```python
from build123d import *

# Parameters (mm, degrees)
CORNERBOSS_EXTRUDE1_DEPTH               = 20
SHELL2_T                                = -3
PUTBACKSHELLBOSS_EXTRUDE1_DEPTH         = 17
TAB_HOLES_SKETCH1_R                     = 1
TABHOLESCUT_EXTRUDE1_DEPTH              = 317.211923597
PADSKETCH3_R                            = 12
PADSKETCH3_R_2                          = 5
PADBOSS_EXTRUDE2_DEPTH                  = 10
STEPPERSHAFTHOLESKETCH4_R               = 5.1
STEPPERSHAFTHOLESKETCH4_R_2             = 1.5
STEPPERSHAFTCUT_EXTRUDE2_DEPTH          = 316.846451025
THREADEDNUTMOUNTHOLESSKETCH5_R          = 1
THREADEDNUTMOUNTHOLESCUT_EXTRUDE4_DEPTH = 10
TRPEGSKETCH1_W                          = 9.8
TRPEGSKETCH1_H                          = 13.9
TRPEGBOSS_EXTRUDE1_DEPTH                = 3.1
TRPEGCAPSKETCH2_W                       = 16
TRPEGCAPSKETCH2_H                       = 17
TRPEGCAPBOSS_EXTRUDE2_DEPTH             = 3
BOTTOMPEGHOLESKETCH3_W                  = 10
BOTTOMPEGHOLESKETCH3_H                  = 13.9
BOTTOMPEGHOLECUT_EXTRUDE1_DEPTH         = 3


with BuildPart() as part:
    # CornerrSketch1 → CornerBoss-Extrude1 (new body)
    with BuildSketch(Plane(origin=(0, 0, 0), x_dir=(1, 0, 0), z_dir=(0, 1, 0))):
        with BuildLine():
            Line((140, 220), (140, 120))
            Line((140, 120), (90, 120))
            Line((90, 120), (90, 0))
            Line((90, 0), (0, 0))
            Line((0, 0), (0, 265.825))
            ThreePointArc((0, 265.825), (17, 282.825), (34, 265.825))
            Line((34, 265.825), (34, 220))
            Line((34, 220), (140, 220))
        make_face()
    extrude(amount=CORNERBOSS_EXTRUDE1_DEPTH)

    # Shell2
    shell2_openings = [part.faces().sort_by_distance(p)[0] for p in [
        (55.952693014, 0, -131.673048366),
    ]]
    offset(amount=SHELL2_T, openings=shell2_openings, kind=Kind.INTERSECTION)

    # PutBackShellSketch2 → PutBackShellBoss-Extrude1 (add)
    with BuildSketch(Plane.XZ.offset(-17)):
        Polygon((67, -3), (87, -3), (87, -123), (137, -123), (137, -143), (67, -143), align=None)
    extrude(amount=PUTBACKSHELLBOSS_EXTRUDE1_DEPTH)

    # Tab holes-Sketch1 → TabHolesCut-Extrude1 (cut, through all)
    with BuildSketch(Plane(origin=(0, 20, 0), x_dir=(1, 0, 0), z_dir=(0, 1, 0))):
        with Locations(Location((120, 130, 0), (0, 0, 270))):
            Circle(TAB_HOLES_SKETCH1_R)
        with Locations(Location((80, 130, 0), (0, 0, 270))):
            Circle(TAB_HOLES_SKETCH1_R)
        with Locations(Location((80, 75, 0), (0, 0, 270))):
            Circle(TAB_HOLES_SKETCH1_R)
        with Locations(Location((80, 20, 0), (0, 0, 270))):
            Circle(TAB_HOLES_SKETCH1_R)
    extrude(amount=-TABHOLESCUT_EXTRUDE1_DEPTH, mode=Mode.SUBTRACT)

    # PadSketch3 → PadBoss-Extrude2 (add)
    with BuildSketch(Plane.XZ.offset(-17)):
        with Locations(Location((17, -265.825, 0), (0, 0, 90))):
            Circle(PADSKETCH3_R)
        with Locations((7, -35)):
            Circle(PADSKETCH3_R_2)
    extrude(amount=PADBOSS_EXTRUDE2_DEPTH)

    # StepperShaftHoleSketch4 → StepperShaftCut-Extrude2 (cut, through all)
    with BuildSketch(Plane.XZ.offset(-7)):
        with Locations(Location((17, -265.825, 0), (0, 0, 270))):
            Circle(STEPPERSHAFTHOLESKETCH4_R)
        with Locations(Location((7, -35, 0), (0, 0, 270))):
            Circle(STEPPERSHAFTHOLESKETCH4_R_2)
    extrude(amount=-STEPPERSHAFTCUT_EXTRUDE2_DEPTH, mode=Mode.SUBTRACT)

    # ThreadedNutMountHolesSketch5 → ThreadedNutMountHolesCut-Extrude4 (cut)
    with BuildSketch(Plane(origin=(0, 7, 0), x_dir=(-1, 0, 0), z_dir=(0, -1, 0))):
        with Locations(Location((-17, 273.825, 0), (0, 0, 90))):
            Circle(THREADEDNUTMOUNTHOLESSKETCH5_R)
        with Locations(Location((-9, 265.825, 0), (0, 0, 90))):
            Circle(THREADEDNUTMOUNTHOLESSKETCH5_R)
        with Locations(Location((-17, 257.825, 0), (0, 0, 90))):
            Circle(THREADEDNUTMOUNTHOLESSKETCH5_R)
        with Locations(Location((-25, 265.825, 0), (0, 0, 90))):
            Circle(THREADEDNUTMOUNTHOLESSKETCH5_R)
    extrude(amount=-THREADEDNUTMOUNTHOLESCUT_EXTRUDE4_DEPTH, mode=Mode.SUBTRACT)

    # TRPegSketch1 → TRPegBoss-Extrude1 (add)
    with BuildSketch(Plane(origin=(140, 0, 0), x_dir=(0, 0, -1), z_dir=(1, 0, 0))):
        with Locations((205, 6.95)):
            Rectangle(TRPEGSKETCH1_W, TRPEGSKETCH1_H)
    extrude(amount=TRPEGBOSS_EXTRUDE1_DEPTH)

    # TRPegCapSketch2 → TRPegCapBoss-Extrude2 (add)
    with BuildSketch(Plane(origin=(143.1, 0, 0), x_dir=(0, 0, -1), z_dir=(1, 0, 0))):
        with Locations((205.1, 8.5)):
            Rectangle(TRPEGCAPSKETCH2_W, TRPEGCAPSKETCH2_H)
    extrude(amount=TRPEGCAPBOSS_EXTRUDE2_DEPTH)

    # BottomPegHoleSketch3 → BottomPegHoleCut-Extrude1 (cut)
    with BuildSketch(Plane.XY):
        with Locations((15, 6.95)):
            Rectangle(BOTTOMPEGHOLESKETCH3_W, BOTTOMPEGHOLESKETCH3_H)
    extrude(amount=-BOTTOMPEGHOLECUT_EXTRUDE1_DEPTH, mode=Mode.SUBTRACT)

    # OverlapChamfer1
    # the kernel refuses this chamfer: 20 mm, written as the material it takes off along each edge
    with BuildSketch(Plane(origin=(90, 20, -120), x_dir=(0.027495876610586317, -0.9996219169112968, 0), z_dir=(0, 0, 1))) as overlapchamfer1_piece_1:
        with BuildLine():
            Line((20.573463904, 0), (-1.130943098, -20.54235587))
            Line((-1.130943098, -20.54235587), (-1.530791864, -20.53135752))
            ThreePointArc((-1.530791864, -20.53135752), (-0.682584541, -10.267956593), (-0.399848767, 0.010998351))
            Line((-0.399848767, 0.010998351), (0.010998351, 0.399848767))
            ThreePointArc((0.010998351, 0.399848767), (10.289953294, 0.117112992), (20.584462254, 0.399848767))
            Line((20.584462254, 0.399848767), (20.573463904, 0))
        make_face()
    extrude(amount=120, mode=Mode.SUBTRACT)
    with BuildSketch(Plane(origin=(140, 20, -120), x_dir=(0, -0.9996219169112968, 0.027495876610586317), z_dir=(-1, 0, 0))) as overlapchamfer1_piece_2:
        with BuildLine():
            Line((20.573463904, 0), (-1.130943098, -20.54235587))
            Line((-1.130943098, -20.54235587), (-1.530791864, -20.53135752))
            ThreePointArc((-1.530791864, -20.53135752), (-0.682584541, -10.267956593), (-0.399848767, 0.010998351))
            Line((-0.399848767, 0.010998351), (0.010998351, 0.399848767))
            ThreePointArc((0.010998351, 0.399848767), (10.289953294, 0.117112992), (20.584462254, 0.399848767))
            Line((20.584462254, 0.399848767), (20.573463904, 0))
        make_face()
    extrude(amount=50, mode=Mode.SUBTRACT)
    with BuildSketch(Plane(origin=(90, 20, -171.433659759), x_dir=(0.027495876610586317, -0.9996219169112968, 0), z_dir=(0, 0, 1))) as overlapchamfer1_piece_3a_section:
        with BuildLine():
            Line((20.573463904, 0), (-1.130943098, -20.54235587))
            Line((-1.130943098, -20.54235587), (-1.530791864, -20.53135752))
            ThreePointArc((-1.530791864, -20.53135752), (-0.682584541, -10.267956593), (-0.399848767, 0.010998351))
            Line((-0.399848767, 0.010998351), (0.010998351, 0.399848767))
            ThreePointArc((0.010998351, 0.399848767), (10.289953294, 0.117112992), (20.584462254, 0.399848767))
            Line((20.584462254, 0.399848767), (20.573463904, 0))
        make_face()
    overlapchamfer1_piece_3a = extrude(amount=171.433659759, mode=Mode.PRIVATE)
    overlapchamfer1_piece_3a = split(overlapchamfer1_piece_3a, bisect_by=Plane(origin=(83.404127464, 13.404127464, -120), z_dir=(0, 0, -1)), keep=Keep.TOP, mode=Mode.PRIVATE)
    with BuildSketch(Plane(origin=(140, 20, -120), x_dir=(0, -0.9996219169112968, 0.027495876610586317), z_dir=(-1, 0, 0))) as overlapchamfer1_piece_3b_section:
        with BuildLine():
            Line((20.573463904, 0), (-1.130943098, -20.54235587))
            Line((-1.130943098, -20.54235587), (-1.530791864, -20.53135752))
            ThreePointArc((-1.530791864, -20.53135752), (-0.682584541, -10.267956593), (-0.399848767, 0.010998351))
            Line((-0.399848767, 0.010998351), (0.010998351, 0.399848767))
            ThreePointArc((0.010998351, 0.399848767), (10.289953294, 0.117112992), (20.584462254, 0.399848767))
            Line((20.584462254, 0.399848767), (20.573463904, 0))
        make_face()
    overlapchamfer1_piece_3b = extrude(amount=101.433659759, mode=Mode.PRIVATE)
    overlapchamfer1_piece_3b = split(overlapchamfer1_piece_3b, bisect_by=Plane(origin=(90, 13.404127464, -126.595872536), z_dir=(-1, 0, 0)), keep=Keep.TOP, mode=Mode.PRIVATE)
    overlapchamfer1_piece_3 = overlapchamfer1_piece_3a & overlapchamfer1_piece_3b
    add(overlapchamfer1_piece_3, mode=Mode.SUBTRACT)


solid = part.part
```
The model under review builds one solid part; all positions refer to its coordinate system, in mm. A direction names the side the tool comes from. Coordinates: 2 decimals unless noted, no trailing zeros. Write each loop counter-clockwise with the first axis right and the second up, starting at its lowest first coordinate (ties: lowest second). Pieces come first, ordered by that corner, then holes.
1) We need section A-A on x = 63. State the section outline as (y, z) points, then the cut area to 3 significant figures.
2) The part is to be moulded in two halves that separate along X. For faces 4 (the face through (34, 10, -243)), 5 (the face through (143.1, 14.3, -205)), 6 (the face through (113, 10, -130)), say which applies: pulls with the +X half, pulls with the -X half, needs draft (parallel to the pull), parting line crosses it, or undercut.
3) We need section B-B on z = -90. State the section outline as (x, y) points, then the cut area to 3 significant figures.
4) Machinability: for faces 1 (the face through (102, 9, -143)), 2 (the face through (67.3, 0, -109.3)), 3 (the face through (86, 10, -220)), which of the approach directions +Z, -Z, +X, -X, +Y, -Y give a long, thin tool a straight path to every point of the face, cutting with its end or side? Answer none if there is none.
5) Clearance check with flat-ended pins moving along their axes: pin 1 Ø2.5 at (x, z) = (17, -273.825) entering from -Y; pin 2 Ø6 at (x, y) = (50.5, 10) entering from -Z; pin 3 Ø6 at (y, z) = (6.5, -170) entering from +X. State where each tip first meets the part, or that it passes through.
6) To check wall thickness, follow probe 1 along X at (y, z) = (3.25, -130); probe 2 along Z at (x, y) = (55.5, 13.5); probe 3 along Z at (x, y) = (120, 5.25). State the ranges of each line that lie inside material, in increasing order.
Answer list:
1. outline: (0, -220) - (20, -220) - (20, 0) - (0, 0) - (0, -3) - (17, -3) - (17, -217) - (0, -217) - close
1. area: 762 mm2
2. face 4: pulls with the +X half
2. face 5: undercut
2. face 6: needs draft
3. outline: (0, 0) - (3, 0) - (3, 17) - (67, 17) - (67, 0) - (90, 0) - (70, 20) - (0, 20) - close
3. area: 512 mm2
4. face 1: -Y
4. face 2: +Z, -Z, +X, -X, -Y
4. face 3: -Z, +X, +Y, -Y
5. pin 1: stops at y = 7
5. pin 2: stops at z = -220
5. pin 3: stops at x = 140
6. probe 1: x = 0 to 3, 67 to 79, 81 to 119, 121 to 140
6. probe 2: z = -220 to -217, -3 to 0
6. probe 3: z = -220 to -217, -143 to -131, -129 to -125.25
